Check sheet for the modelled part. Datum: model origin and axes. Units: mm. A direction names the side the tool comes from. Round coordinates to 2 decimals unless told otherwise and drop trailing zeros. Write each loop counter-clockwise with the first axis right and the second up, starting at its lowest first coordinate (ties: lowest second). Pieces come first, ordered by that corner, then holes. Notation, with made-up numbers: (34.5, 5) - (82.5, 5) arc R21 ccw to (82.5, 17) - close; hole circle Ø2 at (42.25, 7). An arc over 180 degrees is marked (long way). Answer as a JSON object with one key per item and string values. Group by question number.
Item 1: Sectioned sample at C-C on x = 35.5. Record the boundary of the cut face in (y, z), plus the area to 3 significant figures.
Item 2: Set-up check for faces 5 (the flat face through (-1, -6.35, -28)), 6 (the flat face through (1, -3, -1.365)), 7 (the flat face through (0, -15, 5.08)), 8 (the flat face through (-16.381, -3, -16)), 9 (the flat face through (0, -48, 5.08)): record each of +Z, -Z, +X, -X, +Y, -Y from which the full face is reachable in a straight line by a thin tool's end or side.
Item 3: Sectioned sample at B-B on x = -6.5. Record the boundary of the cut face in (y, z), plus the area to 3 significant figures.
Item 4: Thickness scan on line 1 (Z direction, x = -25, y = -34); line 2 (X direction, y = -6, z = -27.5); line 3 (Y direction, x = -45, z = 7). Record the ranges inside material, lowest first.
Item 5: Gauge pin test, flat ends, axial feed: P1, Ø1.9, axis at x = -5, z = 7.5, coming from the -Y side; P2, Ø7, axis at y = -4.5, z = -19, coming from the +X side; P3, Ø1.9, axis at y = -3, z = -13, coming from the -X side; P4, Ø1, axis at x = -11.5, z = -5.5, coming from the +Y side. Record the tip position at first contact, or that the pin passes through.
Item 6: Release check for a two-part mould opening along Z. For faces 1 (the flat face through (0, -3, -31.063)), 2 (the flat face through (17, -3, -16)), 3 (the flat face through (14.958, -3, -14)), 4 (the flat face through (-12.982, -3, -14)) record: pulls with the +Z half, pulls with the -Z half, needs draft (parallel to the pull), parting line crosses it, or undercut.
Item 7: Sectioned sample at A-A on z = -22. Record the boundary of the cut face in (x, y), plus the area to 3 significant figures.
Item 8: Sectioned sample at D-D on y = -9.5. Record the boundary of the cut face in (x, z).
```python
from build123d import *

# Parameters (mm, degrees)
F0_W     = 33.381108
F0_H     = 31.062972
F0_W_2   = 27.94
F0_H_2   = 25.6794
F1_DEPTH = 6.35
F2_DEPTH = 60.452
F3_W     = 111.270344
F3_H     = 4.986666
F4_DEPTH = 3.81


with BuildPart() as f1:
    # F0 (on Front) → F1 (new body)
    with BuildSketch(Plane.XZ):
        with Locations((0.309085, -15.531486)):
            Rectangle(F0_W, F0_H)
        with Locations((0.988458, -14.205176)):
            Rectangle(F0_W_2, F0_H_2, mode=Mode.SUBTRACT)
    extrude(amount=F1_DEPTH)

    # F0 (on Front) → F2 (join)
    with BuildSketch(Plane.XZ):
        Polygon((-55.94426, 5.08), (-55.94426, 0), (-16.381469, 0), (16.999639, 0), (55.326084, 0), (55.326084, 5.08), align=None)
    extrude(amount=F2_DEPTH)

    # F3 (on face) → F4 (join)
    with BuildSketch(Plane.XY.offset(5.08)):
        with Locations((-0.309088, -32.719333)):
            Rectangle(F3_W, F3_H)
    extrude(amount=F4_DEPTH)


solid = f1.part
```
Completed:
{
 "1": {"outline": "(-60.45, 0) - (0, 0) - (0, 5.08) - (-30.23, 5.08) - (-30.23, 8.89) - (-35.21, 8.89) - (-35.21, 5.08) - (-60.45, 5.08) - close", "area": "326 mm²"},
 "2": {"face 5": "-Z, +X, -X, -Y", "face 6": "+Y, -Y", "face 7": "+Z, +X, -X, +Y", "face 8": "-Z, -X, +Y, -Y", "face 9": "+Z, +X, -X, -Y"},
 "3": {"outline": "(-60.45, 0) - (-6.35, 0) - (-6.35, -1.37) - (0, -1.37) - (0, 5.08) - (-30.23, 5.08) - (-30.23, 8.89) - (-35.21, 8.89) - (-35.21, 5.08) - (-60.45, 5.08) - close; (-6.35, -31.06) - (0, -31.06) - (0, -27.04) - (-6.35, -27.04) - close", "area": "360 mm²"},
 "4": {"line 1": "0 to 8.89", "line 2": "-16.38 to 17", "line 3": "-35.21 to -30.23"},
 "5": {"P1": "y = -35.21", "P2": "x = 17", "P3": "x = -16.38", "P4": "through"},
 "6": {"face 1": "pulls with the -Z half", "face 2": "needs draft", "face 3": "undercut", "face 4": "undercut"},
 "7": {"outline": "(-16.38, -6.35) - (-12.98, -6.35) - (-12.98, 0) - (-16.38, 0) - close; (14.96, -6.35) - (17, -6.35) - (17, 0) - (14.96, 0) - close", "area": "34.6 mm²"},
 "8": {"outline": "(-55.94, 0) - (55.33, 0) - (55.33, 5.08) - (-55.94, 5.08) - close"}
}
